Verification items for the finished model (mm, model axes). A direction names the side the tool comes from. Give positions to 0.01 mm unless a question says otherwise; leave off trailing zeros. Loops run counter-clockwise (first coordinate to the right, second up) from the corner with the lowest first, then second, coordinate; pieces in that order, holes last. Notation, with made-up numbers: M 78.25,53.5 L 110.25,53.5 A27 cw 110.25,73.5 Z; hole C 3.5,66.5 d8. An arc over 180 degrees is marked long. Put each result on its own line as item: value. Start each with the question number.
from build123d import *

# Parameters (mm, degrees)
SKETCH1_W           = 30
SKETCH1_H           = 42.7
BOSS_EXTRUDE1_DEPTH = 12.7
SKETCH2_W           = 40
SKETCH2_H           = 12.7
SKETCH2_W_2         = 12.7
SKETCH2_H_2         = 40
SKETCH2_W_3         = 30
CUT_EXTRUDE2_DEPTH  = 12.7


with BuildPart() as part:
    # Sketch1 → Boss-Extrude1 (new body)
    with BuildSketch(Plane(origin=(0, 0, 0), x_dir=(1, 0, 0), z_dir=(0, 1, 0))):
        Polygon((140.4, 150), (-140.4, 150), (-140.4, 107.3), (-140.4, -107.3), (-140.4, -150), (140.4, -150), (140.4, -107.3), (140.4, 107.3), align=None)
        with Locations((-155.4, 128.65)):
            Rectangle(SKETCH1_W, SKETCH1_H)
        with Locations((155.4, 128.65)):
            Rectangle(SKETCH1_W, SKETCH1_H)
        with Locations((-155.4, -128.65)):
            Rectangle(SKETCH1_W, SKETCH1_H)
        with Locations((155.4, -128.65)):
            Rectangle(SKETCH1_W, SKETCH1_H)
    extrude(amount=BOSS_EXTRUDE1_DEPTH)

    # Sketch2 → Cut-Extrude2 (cut)
    with BuildSketch(Plane(origin=(0, 12.7, 0), x_dir=(1, 0, 0), z_dir=(0, 1, 0))):
        with Locations((0, -143.65)):
            Rectangle(SKETCH2_W, SKETCH2_H)
        with Locations((-134.05, 0)):
            Rectangle(SKETCH2_W_2, SKETCH2_H_2)
        with Locations((134.05, 0)):
            Rectangle(SKETCH2_W_2, SKETCH2_H_2)
        with Locations((0, 143.65)):
            Rectangle(SKETCH2_W, SKETCH2_H)
        with Locations((-155.4, 143.65)):
            Rectangle(SKETCH2_W_3, SKETCH2_H)
        with Locations((155.4, 143.65)):
            Rectangle(SKETCH2_W_3, SKETCH2_H)
        with Locations((-155.4, -143.65)):
            Rectangle(SKETCH2_W_3, SKETCH2_H)
        with Locations((155.4, -143.65)):
            Rectangle(SKETCH2_W_3, SKETCH2_H)
    extrude(amount=-CUT_EXTRUDE2_DEPTH, mode=Mode.SUBTRACT)


solid = part.part
Q1. Cross-section at C-C, the plane x = -10. Record the boundary of the cut face in (y, z), then the cut area to 3 significant figures.
Q2. Cross-section at B-B, the plane z = 90. Record the boundary of the cut face in (x, y).
Q3. Release check for a two-part mould opening along Z. For faces 6 (the face through (155, 6, 137.3)), 7 (the face through (-156, 6, 107.3)), 8 (the face through (-170.4, 6, 123)) record: pulls with the +Z half, pulls with the -Z half, needs draft (parallel to the pull), parting line crosses it, or undercut.
Q4. Scan lines: L1, parallel to X at y = 5, z = 27; L2, parallel to Z at x = -157, y = 2; L3, parallel to X at y = 7, z = 19.5. Record each from-to range of solid material in increasing order.
Q5. Cross-section at A-A, the plane x = -149. Record the boundary of the cut face in (y, z), then the cut area to 3 significant figures.
Q6. Go/stop test with flat-tipped pins: pin 1 (1 mm diameter, centred on y = 4.5, z = -22.5, fed in from -X); pin 2 (4 mm diameter, centred on y = 4.5, z = 2.5, fed in from +X); pin 3 (4 mm diameter, centred on x = 157.5, y = 6.5, fed in from +Z). Record where each tip stops, or that it passes through.
Q7. Set-up check for faces 1 (the face through (-156, 6, -107.3)), 2 (the face through (155, 6, -137.3)), 3 (the face through (20, 6, -144)), 4 (the face through (134, 6, -20)), 5 (the face through (0, 6, 137.3)): record each of +Z, -Z, +X, -X, +Y, -Y from which the full face is reachable in a straight line by a thin tool's end or side.
Ans:
1. outline: M 0,-137.3 L 12.7,-137.3 L 12.7,137.3 L 0,137.3 Z
1. area: 3,490 mm^2
2. outline: M -140.4,0 L 140.4,0 L 140.4,12.7 L -140.4,12.7 Z
3. face 6: pulls with the +Z half
3. face 7: undercut
3. face 8: needs draft
4. L1: x = -140.4 to 140.4
4. L2: z = -137.3 to -107.3, 107.3 to 137.3
4. L3: x = -127.7 to 127.7
5. outline: M 0,-137.3 L 12.7,-137.3 L 12.7,-107.3 L 0,-107.3 Z; M 0,107.3 L 12.7,107.3 L 12.7,137.3 L 0,137.3 Z
5. area: 762 mm^2
6. pin 1: stops at x = -140.4
6. pin 2: stops at x = 127.7
6. pin 3: stops at z = 137.3
7. face 1: -X, +Y, -Y
7. face 2: -Z, +X, +Y, -Y
7. face 3: -Z, +Y, -Y
7. face 4: +X, +Y, -Y
7. face 5: +Z, +Y, -Y
